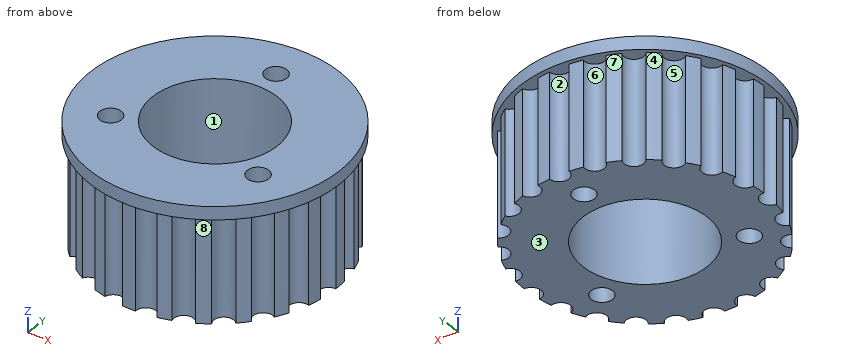
```python
from build123d import *

# Parameters (mm, degrees)
SKETCH_1_R          = 9.5
EXTRUDE_1_DEPTH     = 16
SKETCH_2_R          = 19
SKETCH_2_R_2        = 9.5
EXTRUDE_2_DEPTH     = 2
SKETCH_4_R          = 1.65
CUT_EXTRUDE_1_DEPTH = 19


with BuildPart() as part:
    # Эскиз1 → Бобышка-Вытянуть1 (new body)
    with BuildSketch(Plane.XY):
        with BuildLine():
            ThreePointArc((-1.498740142, 18.241534666), (-2.492258178, 18.13252487), (-3.478344362, 17.969444329))
            ThreePointArc((-3.478344362, 17.969444329), (-4.533395146, 16.179899179), (-6.364669946, 17.160733827))
            ThreePointArc((-6.364669946, 17.160733827), (-7.291935147, 16.787718451), (-8.197455977, 16.364642511))
            ThreePointArc((-8.197455977, 16.364642511), (-8.730569112, 14.356809255), (-10.758561296, 14.807199865))
            ThreePointArc((-10.758561296, 14.807199865), (-11.550802645, 14.197843754), (-12.308599783, 13.54615002))
            ThreePointArc((-12.308599783, 13.54615002), (-12.280236708, 11.468940466), (-14.354539373, 11.355483627))
            ThreePointArc((-14.354539373, 11.355483627), (-14.952999952, 10.554979936), (-15.506871051, 9.723001553))
            ThreePointArc((-15.506871051, 9.723001553), (-14.919135325, 7.730472829), (-16.885906931, 7.061583116))
            ThreePointArc((-16.885906931, 7.061583116), (-17.246201658, 6.129301542), (-17.555068633, 5.17874254))
            ThreePointArc((-17.555068633, 5.17874254), (-16.451549925, 3.418671387), (-18.164924021, 2.243957291))
            ThreePointArc((-18.164924021, 2.243957291), (-18.260331482, 1.249040892), (-18.301287083, 0.250399884))
            ThreePointArc((-18.301287083, 0.250399884), (-16.763828329, -1.146677272), (-18.096731795, -2.740092582))
            ThreePointArc((-18.096731795, -2.740092582), (-17.920176057, -3.723855407), (-17.690182793, -4.696513786))
            ThreePointArc((-17.690182793, -4.696513786), (-15.832810274, -5.626982123), (-16.686387758, -7.520922323))
            ThreePointArc((-16.686387758, -7.520922323), (-16.250963152, -8.420570386), (-15.767078573, -9.295108514))
            ThreePointArc((-15.767078573, -9.295108514), (-13.727545112, -9.689959452), (-14.038490677, -11.743959661))
            ThreePointArc((-14.038490677, -11.743959661), (-13.376490654, -12.49277018), (-12.674602264, -13.204327565))
            ThreePointArc((-12.674602264, -13.204327565), (-10.604170729, -13.034276818), (-10.349422964, -15.096001236))
            ThreePointArc((-10.349422964, -15.096001236), (-9.509945037, -15.638438361), (-8.642108688, -16.134242047))
            ThreePointArc((-8.642108688, -16.134242047), (-6.694333513, -15.411901499), (-5.892785895, -17.328441459))
            ThreePointArc((-5.892785895, -17.328441459), (-4.938090302, -17.62427511), (-3.968669445, -17.867553605))
            ThreePointArc((-3.968669445, -17.867553605), (-2.288008205, -16.646495951), (-0.999107855, -18.275710451))
            ThreePointArc((-0.999107855, -18.275710451), (0, -18.303), (0.999107855, -18.275710451))
            ThreePointArc((0.999107855, -18.275710451), (2.288008205, -16.646495951), (3.968669445, -17.867553605))
            ThreePointArc((3.968669445, -17.867553605), (4.938090302, -17.62427511), (5.892785895, -17.328441459))
            ThreePointArc((5.892785895, -17.328441459), (6.694333513, -15.411901499), (8.642108688, -16.134242047))
            ThreePointArc((8.642108688, -16.134242047), (9.509945037, -15.638438361), (10.349422964, -15.096001236))
            ThreePointArc((10.349422964, -15.096001236), (10.604170729, -13.034276818), (12.674602264, -13.204327565))
            ThreePointArc((12.674602264, -13.204327565), (13.376490654, -12.49277018), (14.038490677, -11.743959661))
            ThreePointArc((14.038490677, -11.743959661), (13.727545112, -9.689959452), (15.767078573, -9.295108514))
            ThreePointArc((15.767078573, -9.295108514), (16.250963152, -8.420570386), (16.686387758, -7.520922323))
            ThreePointArc((16.686387758, -7.520922323), (15.832810274, -5.626982123), (17.690182793, -4.696513786))
            ThreePointArc((17.690182793, -4.696513786), (17.920176057, -3.723855407), (18.096731795, -2.740092582))
            ThreePointArc((18.096731795, -2.740092582), (16.763828329, -1.146677272), (18.301287083, 0.250399884))
            ThreePointArc((18.301287083, 0.250399884), (18.260331482, 1.249040892), (18.164924021, 2.243957291))
            ThreePointArc((18.164924021, 2.243957291), (16.451549925, 3.418671387), (17.555068633, 5.17874254))
            ThreePointArc((17.555068633, 5.17874254), (17.246201658, 6.129301542), (16.885906931, 7.061583116))
            ThreePointArc((16.885906931, 7.061583116), (14.919135325, 7.730472829), (15.506871051, 9.723001553))
            ThreePointArc((15.506871051, 9.723001553), (14.952999952, 10.554979936), (14.354539373, 11.355483627))
            ThreePointArc((14.354539373, 11.355483627), (12.280236708, 11.468940466), (12.308599783, 13.54615002))
            ThreePointArc((12.308599783, 13.54615002), (11.550802645, 14.197843754), (10.758561296, 14.807199865))
            ThreePointArc((10.758561296, 14.807199865), (8.730569112, 14.356809255), (8.197455977, 16.364642511))
            ThreePointArc((8.197455977, 16.364642511), (7.291935147, 16.787718451), (6.364669946, 17.160733827))
            ThreePointArc((6.364669946, 17.160733827), (4.533395146, 16.179899179), (3.478344362, 17.969444329))
            ThreePointArc((3.478344362, 17.969444329), (2.492258178, 18.13252487), (1.498740142, 18.241534666))
            ThreePointArc((1.498740142, 18.241534666), (0, 16.803), (-1.498740142, 18.241534666))
        make_face()
        Circle(SKETCH_1_R, mode=Mode.SUBTRACT)
    extrude(amount=EXTRUDE_1_DEPTH)

    # Эскиз2 → Бобышка-Вытянуть2 (add)
    with BuildSketch(Plane.XY.offset(16)):
        Circle(SKETCH_2_R)
        Circle(SKETCH_2_R_2, mode=Mode.SUBTRACT)
    extrude(amount=EXTRUDE_2_DEPTH)

    # Эскиз4 → Вырез-Вытянуть1 (cut, through all)
    with BuildSketch(Plane.XY.offset(18)):
        with Locations((0, 13)):
            Circle(SKETCH_4_R)
        with Locations((11.258330249, -6.5)):
            Circle(SKETCH_4_R)
        with Locations((-11.258330249, -6.5)):
            Circle(SKETCH_4_R)
    extrude(amount=-CUT_EXTRUDE_1_DEPTH, mode=Mode.SUBTRACT)


solid = part.part
```
The model under review builds one solid part; all positions refer to its coordinate system, in mm. Face numbers are marked on the shaded views. A direction names the side the tool comes from. Coordinates: 2 decimals unless noted, no trailing zeros. Order: outer loops, then holes, each group sorted by start corner. A loop starts at its lowest first (then second) coordinate and runs counter-clockwise, first axis right, second up. Notation, with made-up numbers: (-26, 69) -> (7, 69) arc R24 ccw to (7, 81) -> close; hole circle Ø2 at (77, -11). An arc over 180 degrees is marked (long way). Answer in a Markdown table with one row per item. Add a question column.
Item 1: We need section C-C on y = -6.5. Write out the cut boundary in (x, z), plus the area to 3 significant figures.
Item 2: Mouldability with a two-part tool opening along X and no side actions: class the marked faces 6, 7 and 8 as +X half, -X half, draft (parallel to the pull), parting line (faces both ways), or undercut.
Item 3: We need section B-B on x = 0. Write out the cut boundary in (y, z).
Item 4: We need section D-D on z = 9.75. Give the number of separate pieces and of enclosed holes in the cut face, plus the area to 3 significant figures.
Item 5: To check wall thickness, follow probe 1 along Z at (x, y) = (-10.5, -15); probe 2 along X at (y, z) = (-1, 2.5); probe 3 along Y at (x, z) = (-6, 1.25). State the ranges of each line that lie inside material, in increasing order.
Item 6: We need section A-A on y = 3. Write out the cut boundary in (x, z).
Item 7: Clearance check with flat-ended pins moving along their axes: pin 1 (6 mm diameter, centred on x = 15, z = 7, fed in from -Y); pin 2 (1.5 mm diameter, centred on x = 6, z = 3, fed in from +Y); pin 3 (6 mm diameter, centred on x = -9.5, z = 11.5, fed in from -Y); pin 4 (2 mm diameter, centred on x = -11.26, y = -6.5, fed in from -Z). State where each tip first meets the part, or that it passes through.
Item 8: Machinability: for the marked faces 1, 2, 3, 4 and 5, which of the approach directions +Z, -Z, +X, -X, +Y, -Y give a long, thin tool a straight path to every point of the face, cutting with its end or side? Answer none if there is none.
Final values:
| question | item | result |
|---|---|---|
| 1 | outline | (-17.85, 16) -> (-15.79, 16) -> (-15.79, 0) -> (-12.91, 0) -> (-12.91, 18) -> (-17.85, 18) -> close; (-9.61, 0) -> (-6.93, 0) -> (-6.93, 18) -> (-9.61, 18) -> close; (6.93, 0) -> (9.61, 0) -> (9.61, 18) -> (6.93, 18) -> close; (12.91, 0) -> (15.79, 0) -> (15.79, 16) -> (17.85, 16) -> (17.85, 18) -> (12.91, 18) -> close |
| 1 | area | 209 mm2 |
| 2 | face 6 | undercut |
| 2 | face 7 | -X half |
| 2 | face 8 | +X half |
| 3 | outline | (-19, 16) -> (-18.3, 16) -> (-18.3, 0) -> (-9.5, 0) -> (-9.5, 18) -> (-19, 18) -> close; (9.5, 0) -> (11.35, 0) -> (11.35, 18) -> (9.5, 18) -> close; (14.65, 0) -> (16.8, 0) -> (16.8, 16) -> (19, 16) -> (19, 18) -> (14.65, 18) -> close |
| 4 | separate pieces | 1 |
| 4 | enclosed holes | 4 |
| 4 | area | 663 mm2 |
| 5 | probe 1 | z = 16 to 18 |
| 5 | probe 2 | x = -16.78 to -9.45, 9.45 to 16.78 |
| 5 | probe 3 | y = -16.03 to -7.37, 7.37 to 16.56 |
| 6 | outline | (-18.76, 16) -> (-16.61, 16) -> (-16.61, 0) -> (-9.01, 0) -> (-9.01, 18) -> (-18.76, 18) -> close; (9.01, 0) -> (16.61, 0) -> (16.61, 16) -> (18.76, 16) -> (18.76, 18) -> (9.01, 18) -> close |
| 7 | pin 1 | stops at y = -13.2 |
| 7 | pin 2 | stops at y = 17.16 |
| 7 | pin 3 | stops at y = -16.13 |
| 7 | pin 4 | passes through |
| 8 | face 1 | +Z, -Z |
| 8 | face 2 | -Z, +Y |
| 8 | face 3 | -Z, +X, -X, +Y, -Y |
| 8 | face 4 | -Z, -X, +Y |
| 8 | face 5 | -Z |
